Source: CAD feature listing. Evaluate the final solid. Frame: model axes, mm. A direction names the side the tool comes from. Round coordinates to 2 decimals unless told otherwise and drop trailing zeros. Write each loop counter-clockwise with the first axis right and the second up, starting at its lowest first coordinate (ties: lowest second). Pieces come first, ordered by that corner, then holes. Notation, with made-up numbers: M 6,-12 L 45,-12 A30 ccw 45,18 Z; hole C 50,20 d4. An arc over 180 degrees is marked long. Answer in a Markdown table with one row per item.
from build123d import *

# Parameters (mm, degrees)
SKETCH1_W           = 45
SKETCH1_H           = 15
BOSS_EXTRUDE1_DEPTH = 8
SKETCH2_W           = 30
SKETCH2_H           = 15
BOSS_EXTRUDE2_DEPTH = 18
FILLET1_R           = 2
SKETCH3_R           = 1.5
CUT_EXTRUDE1_DEPTH  = 20
CHAMFER1_SIZE       = 1
SKETCH13_R          = 12.2
CUT_EXTRUDE4_DEPTH  = 20
SKETCH14_W          = 24.4
SKETCH14_H          = 5
CUT_EXTRUDE5_DEPTH  = 20
FILLET4_R           = 1


with BuildPart() as part:
    # Sketch1 → Boss-Extrude1 (new body)
    with BuildSketch(Plane(origin=(0, 0, 0), x_dir=(1, 0, 0), z_dir=(0, 1, 0))):
        with Locations((22.5, 7.5)):
            Rectangle(SKETCH1_W, SKETCH1_H)
    extrude(amount=BOSS_EXTRUDE1_DEPTH)

    # Sketch2 → Boss-Extrude2 (add)
    with BuildSketch(Plane(origin=(0, 8, 0), x_dir=(1, 0, 0), z_dir=(0, 1, 0))):
        with Locations((22.5, 7.5)):
            Rectangle(SKETCH2_W, SKETCH2_H)
    extrude(amount=BOSS_EXTRUDE2_DEPTH)

    # Fillet1
    fillet1_edges = [part.edges().sort_by_distance(p)[0] for p in [
        (7.5, 8, -7.5),
        (37.5, 8, -7.5),
        (0, 4, 0),
        (0, 4, -15),
        (45, 4, -15),
        (45, 4, 0),
    ]]
    fillet(fillet1_edges, radius=FILLET1_R)

    # Sketch3 → Cut-Extrude1 (cut)
    with BuildSketch(Plane(origin=(0, 8, 0), x_dir=(1, 0, 0), z_dir=(0, 1, 0))):
        with Locations(Location((3, 7.524826623, 0), (0, 0, 270))):
            Circle(SKETCH3_R)
        with Locations(Location((42, 7.524826623, 0), (0, 0, 270))):
            Circle(SKETCH3_R)
    extrude(amount=-CUT_EXTRUDE1_DEPTH, mode=Mode.SUBTRACT)

    # Chamfer1
    chamfer1_edges = [part.edges().sort_by_distance(p)[0] for p in [
        (3, 8, -9.024826623),
        (42, 8, -9.024826623),
    ]]
    chamfer(chamfer1_edges, length=CHAMFER1_SIZE - 0.0001)  # a hair under: the kernel refuses the full size

    # Sketch13 → Cut-Extrude4 (cut)
    with BuildSketch(Plane.XY):
        with Locations((22.484903529, 21)):
            Circle(SKETCH13_R)
    extrude(amount=-CUT_EXTRUDE4_DEPTH, mode=Mode.SUBTRACT)

    # Sketch14 → Cut-Extrude5 (cut)
    with BuildSketch(Plane.XY):
        with Locations((22.484903529, 23.5)):
            Rectangle(SKETCH14_W, SKETCH14_H)
    extrude(amount=-CUT_EXTRUDE5_DEPTH, mode=Mode.SUBTRACT)

    # Fillet4
    fillet4_edges = [part.edges().sort_by_distance(p)[0] for p in [
        (22.484903529, 8.8, 0),
        (22.484903529, 8.8, -15),
        (10.284903529, 23.5, -15),
        (10.284903529, 26, -7.5),
        (34.684903529, 23.5, -15),
        (34.684903529, 26, -7.5),
        (10.284903529, 23.5, 0),
        (34.684903529, 23.5, 0),
    ]]
    fillet(fillet4_edges, radius=FILLET4_R)


solid = part.part
Q1. Section C-C (z = -11.25). Return loops of the section in (x, y), and give its area (3 significant figures).
Solutions:
| item | result |
|---|---|
| outline | M 0,0 L 45,0 L 45,8 L 39.5,8 A2 cw 37.5,10 L 37.5,26 L 35.68,26 A1 ccw 34.68,25 L 34.68,21 A12.2 cw 10.28,21 L 10.28,25 A1 ccw 9.28,26 L 7.5,26 L 7.5,10 A2 cw 5.5,8 L 0,8 Z |
| area | 545 mm2 |
Q2. Pull-direction query (X, two-part tool) for faces 5 (the flat face through (37.5, 18, -7)), 6 (the cylindrical face through (10, 23.5, -14.7)), 7 (the flat face through (37, 26, -8)); classes: pulls with the +X half, pulls with the -X half, needs draft (parallel to the pull), parting line crosses it, or undercut.
Solutions:
| item | result |
|---|---|
| face 5 | pulls with the +X half |
| face 6 | undercut |
| face 7 | needs draft |
Q3. Section D-D (y = 4.75). Return loops of the section in (x, z), and give its area (3 significant figures).
Solutions:
| item | result |
|---|---|
| outline | M 0,-13 A2 ccw 2,-15 L 43,-15 A2 ccw 45,-13 L 45,-2 A2 ccw 43,0 L 2,0 A2 ccw 0,-2 Z; hole C 3,-7.52 d3; hole C 42,-7.52 d3 |
| area | 657 mm2 |
Q4. Contact query for flat-ended pins moving along their axis: pin 1 Ø2 at (x, z) = (32.5, -13) entering from -Y; pin 2 Ø4.5 at (y, z) = (19, -7.5) entering from -X; pin 3 Ø5 at (y, z) = (14.5, -11) entering from +X; pin 4 Ø1 at (x, z) = (32.5, -9) entering from +Y. Output: stop coordinate, or through.
Solutions:
| item | result |
|---|---|
| pin 1 | stops at y = 0 |
| pin 2 | stops at x = 7.5 |
| pin 3 | stops at x = 37.5 |
| pin 4 | stops at y = 14.81 |
Q5. Section A-A (x = 42). Return loops of the section in (y, z).
Solutions:
| item | result |
|---|---|
| outline | M 0,-15 L 8,-15 L 8,-10.02 L 7,-9.02 L 0,-9.02 Z; M 0,-6.02 L 7,-6.02 L 8,-5.02 L 8,0 L 0,0 Z |
Q6. Material intervals for probe 1 along X at (y, z) = (20.75, -6.75); probe 2 along Y at (x, z) = (22.5, -12.25); probe 3 along X at (y, z) = (17.5, -8.75), sorted ascending.
Solutions:
| item | result |
|---|---|
| probe 1 | x = 7.5 to 10.29, 34.68 to 37.5 |
| probe 2 | y = 0 to 8.8 |
| probe 3 | x = 7.5 to 10.8, 34.17 to 37.5 |
Q7. Section B-B (y = 21.75). Return loops of the section in (x, z), and give its area (3 significant figures).
Solutions:
| item | result |
|---|---|
| outline | M 7.5,-15 L 9.28,-15 A1 ccw 10.28,-14 L 10.28,-1 A1 ccw 9.28,0 L 7.5,0 Z; M 34.68,-14 A1 ccw 35.68,-15 L 37.5,-15 L 37.5,0 L 35.68,0 A1 ccw 34.68,-1 Z |
| area | 83.1 mm2 |
Q8. Access query for faces 1 (the cylindrical face through (10, 25.7, -7.6)), 2 (the cylindrical face through (10, 23.5, -0.3)), 3 (the flat face through (7.5, 18, -7)), 4 (the cylindrical face through (34.986, 23.535, -14.715)). Directions: +Z, -Z, +X, -X, +Y, -Y. A direction counts if a zero-diameter tool reaches every point of the face in a straight line with its end or side. Return the directions, or none.
Solutions:
| item | result |
|---|---|
| face 1 | +Z, -Z, +Y |
| face 2 | +Z, +Y |
| face 3 | +Z, -Z, -X, +Y |
| face 4 | -Z, +Y |
